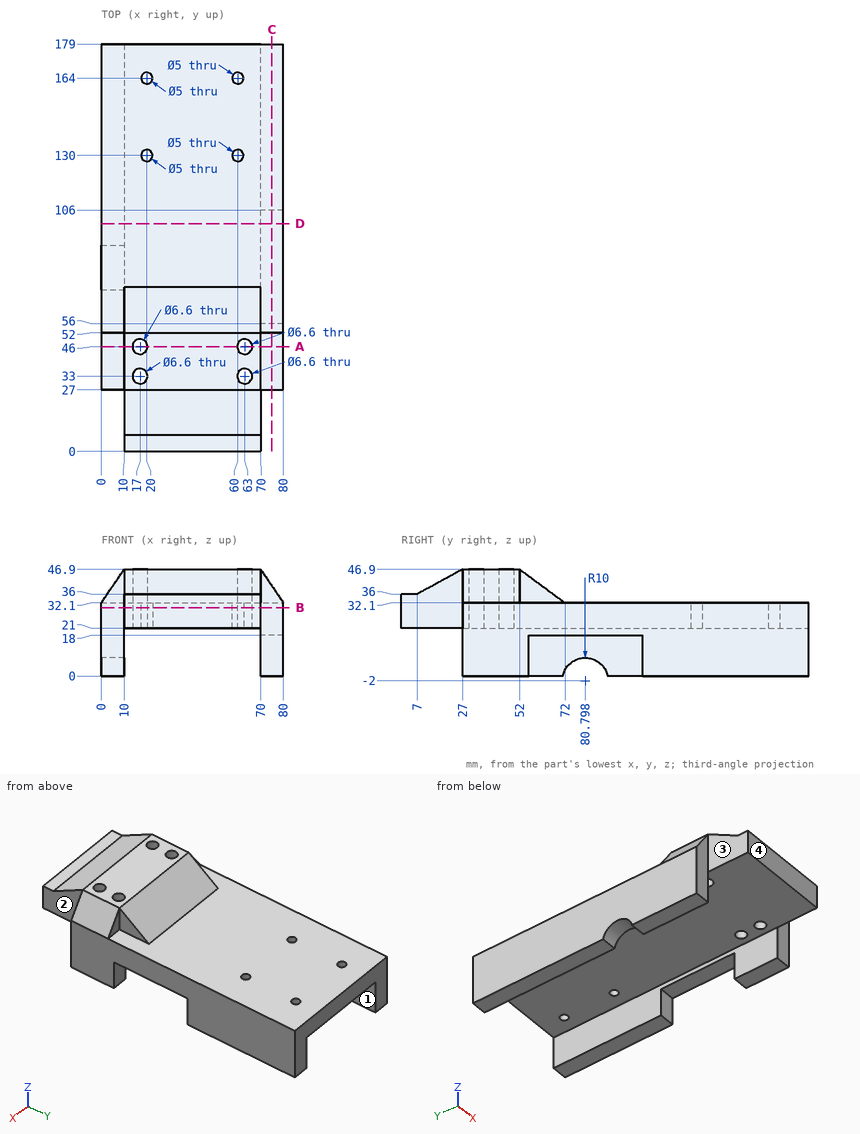
For this review, use the dimensioned drawing (mm, ordinates from the lowest corner) and the shaded views. A direction names the side the tool comes from. Round coordinates to 2 decimals unless told otherwise and drop trailing zeros. Write each loop counter-clockwise with the first axis right and the second up, starting at its lowest first coordinate (ties: lowest second). Pieces come first, ordered by that corner, then holes. Notation, with made-up numbers: M 1.5,60 L 25.5,60 A34 ccw 25.5,98 Z; hole C 71,20 d9. An arc over 180 degrees is marked long. Use CSV: the item, a comma, the result in double quotes. Start each with the question number.
(1) Clearance check with flat-ended pins moving along their axes: P1, Ø5, axis at x = 76, z = 42, coming from the +Y side; P2, Ø7.5, axis at x = 53.5, y = 4.5, coming from the +Z side; P3, Ø6, axis at x = 60, y = 130, coming from the -Z side. State where each tip first meets the part, or that it passes through.
(2) Tool access review of the marked faces 1, 2, 3 and 4: name each direction out of +Z, -Z, +X, -X, +Y, -Y from which nothing blocks a thin tool from reaching the whole face with its end or side.
(3) We need section C-C, the plane x = 75. State the section outline as (y, z) points.
(4) We need section D-D, the plane y = 100. State the section outline as (x, z) points.
(5) We need section B-B, the plane z = 30. State how many separate pieces and enclosed holes the cut face has, then the cut area to 3 significant figures.
(6) For line 1 along Y through (x, z) = (63, 29); line 2 along X through (y, z) = (164, 27.75); line 3 along Y through (x, z) = (77, 10.5), list the stretches that pass through material, from the lowest coordinate up.
(7) We need section A-A, the plane y = 46. State the section outline as (x, z) points, then the cut area to 3 significant figures.
Findings:
1,P1,"y = 52"
1,P2,"z = 36.68"
1,P3,"z = 21"
2,face 1,"-Z, +Y, -Y"
2,face 2,"+Z, -Z, +X, -Y"
2,face 3,"+Z, -Z, -X, -Y"
2,face 4,"+Z, -Z, +X, -X, -Y"
3,outline,"M 27,0 L 56,0 L 56,18 L 106,18 L 106,0 L 179,0 L 179,32.1 L 52,32.1 L 52,39.5 L 27,39.5 Z"
4,outline,"M 0,0 L 10,0 L 10,21 L 70,21 L 70,18 L 80,18 L 80,32.1 L 0,32.1 Z"
5,separate pieces,"1"
5,enclosed holes,"8"
5,area,"13,600 mm^2"
6,line 1,"0 to 29.7, 36.3 to 42.7, 49.3 to 179"
6,line 2,"0 to 17.5, 22.5 to 57.5, 62.5 to 80"
6,line 3,"27 to 56, 106 to 179"
7,outline,"M 0,0 L 10,0 L 10,21 L 13.7,21 L 13.7,46.9 L 10,46.9 L 0,32.1 Z; M 20.3,21 L 59.7,21 L 59.7,46.9 L 20.3,46.9 Z; M 66.3,21 L 70,21 L 70,0 L 80,0 L 80,32.1 L 70,46.9 L 66.3,46.9 Z"
7,area,"2,000 mm^2"
